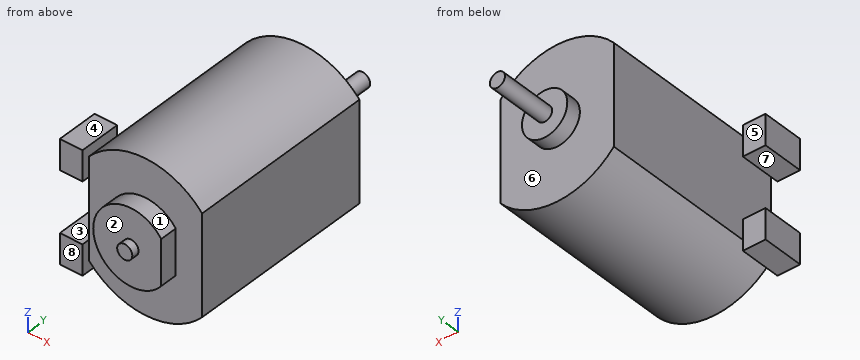
from build123d import *

# Parameters (mm, degrees)
SKETCH_1_R            = 10
EXTRUDE_1_DEPTH       = 25
CUT_EXTRUDE_2_1_REACH = 30.723
SKETCH_2_W            = 2.5
SKETCH_2_H            = 20
SKETCH_3_R            = 3
EXTRUDE_2_DEPTH       = 2
EXTRUDE_START         = -2
SKETCH_4_R            = 1
EXTRUDE_3_DEPTH       = 9.5
EXTRUDE_START_2       = -25
EXTRUDE_4_DEPTH       = 27.3
EXTRUDE_START_3       = 1
SKETCH_6_R            = 1
EXTRUDE_5_DEPTH       = 1
EXTRUDE_6_DEPTH       = 3


with BuildPart() as part:
    # 草图1 → 圆柱凸台-拉伸1 (new body)
    with BuildSketch(Plane(origin=(0, 0, 0), x_dir=(1, 0, 0), z_dir=(0, 1, 0))):
        with Locations(Location((0, 0, 0), (0, 0, 270))):
            Circle(SKETCH_1_R)
    extrude(amount=EXTRUDE_1_DEPTH)

    # 草图2 → 2边切除切除-拉伸1 (cut, up to next)
    with BuildSketch(Plane.XZ, mode=Mode.PRIVATE) as cut_extrude_2_1_sk1:
        with Locations((-8.75, 0)):
            Rectangle(SKETCH_2_W, SKETCH_2_H)
    cut_extrude_2_1_tool1 = extrude(cut_extrude_2_1_sk1.sketch, amount=-CUT_EXTRUDE_2_1_REACH, mode=Mode.PRIVATE) & part.part
    # 草图2 → 2边切除切除-拉伸1 (cut, up to next)
    with BuildSketch(Plane.XZ, mode=Mode.PRIVATE) as cut_extrude_2_1_sk2:
        with Locations((8.75, 0)):
            Rectangle(SKETCH_2_W, SKETCH_2_H)
    cut_extrude_2_1_tool2 = extrude(cut_extrude_2_1_sk2.sketch, amount=-CUT_EXTRUDE_2_1_REACH, mode=Mode.PRIVATE) & part.part
    add(cut_extrude_2_1_tool1.solids().sort_by_distance((-8.75, 0, 0))[0], mode=Mode.SUBTRACT)
    add(cut_extrude_2_1_tool2.solids().sort_by_distance((8.75, 0, 0))[0], mode=Mode.SUBTRACT)

    # 草图3 → 前转凸台-拉伸2 (add)
    with BuildSketch(Plane(origin=(0, 25, 0), x_dir=(1, 0, 0), z_dir=(0, 1, 0))):
        with Locations(Location((0, 0, 0), (0, 0, 270))):
            Circle(SKETCH_3_R)
    extrude(amount=EXTRUDE_2_DEPTH)

    # 草图4 → 前转杆凸台-拉伸3 (add)
    with BuildSketch(Plane(origin=(0, 27, 0), x_dir=(1, 0, 0), z_dir=(0, 1, 0)).offset(EXTRUDE_START)):
        with Locations(Location((0, 0, 0), (0, 0, 270))):
            Circle(SKETCH_4_R)
    extrude(amount=EXTRUDE_3_DEPTH)

    # 草图5 → 后转凸台-拉伸4 (add)
    with BuildSketch(Plane.XZ.offset(EXTRUDE_START_2)):
        with BuildLine():
            Line((4, 3), (4, -3))
            ThreePointArc((4, -3), (-5, 0), (4, 3))
        make_face()
    extrude(amount=EXTRUDE_4_DEPTH)

    # 草图6 → 后转杆凸台-拉伸5 (add)
    with BuildSketch(Plane.XZ.offset(2.3).offset(EXTRUDE_START_3)):
        with Locations(Location((0, 0, 0), (0, 0, 90))):
            Circle(SKETCH_6_R)
    extrude(amount=-EXTRUDE_5_DEPTH)

    # 草图7 → 引线凸台-拉伸6 (add)
    with BuildSketch(Plane.ZY.offset(7.5)):
        Polygon((-8, 3), (-8, 4.5), (-4, 4.5), (-4, 3), (-4, -1), (-8, -1), align=None)
        Polygon((8, 3), (8, -1), (4, -1), (4, 3), (4, 4.5), (8, 4.5), align=None)
    extrude(amount=EXTRUDE_6_DEPTH)


solid = part.part
Input: part model. Units: mm. Frame: model coordinates. Face numbers are marked on the shaded views. A direction names the side the tool comes from. Round coordinates to 2 decimals unless told otherwise and drop trailing zeros. Order: outer loops, then holes, each group sorted by start corner. A loop starts at its lowest first (then second) coordinate and runs counter-clockwise, first axis right, second up. Notation, with made-up numbers: (34.25, 81.5) - (78.25, 81.5) arc R19 ccw to (78.25, 117.5) - close; hole circle Ø8 at (83.25, 50.5). An arc over 180 degrees is marked (long way). Answer as a JSON object with one key per item and string values. Group by question number.
(1) Material intervals for probe 1 along Y at (x, z) = (-4, -1.5); probe 2 along Y at (x, z) = (4.5, 7.75); probe 3 along X at (y, z) = (22.5, 3), sorted ascending. Write a range as from..to.
(2) Cut plane A-A (x = -9). Return loops of the section in (y, z), then the cut area to 3 significant figures.
(3) Pin query (flat end, axial travel): P1, Ø0.9, axis at x = -9, z = 7, coming from the -Y side; P2, Ø8, axis at x = 5.5, y = 28, coming from the -Z side; P3, Ø7, axis at x = 1, z = 1.5, coming from the -Y side; P4, Ø3, axis at x = -5.5, y = 12.5, coming from the -Z side. Return the tip coordinate at first contact, or that it passes through.
(4) Reachability of the marked faces 4, 5, 6, 7 and 8 from +Z, -Z, +X, -X, +Y, -Y: full face, straight path, thin tool, end or side. Return the list, or none.
(5) Draft query along Z for the marked faces 1, 2 and 3. Return one class per face: released by +Z, released by -Z, zero draft, split by the parting line, or undercut.
(6) Cut plane C-C (z = 0). Return loops of the section in (x, y).
(7) Cut plane B-B (y = 2). Return loops of the section in (x, z).
(8) Cut plane D-D (x = 1.75). Return loops of the section in (y, z), then the cut area to 3 significant figures.
Here are the results:
{
 "1": {"probe 1": "y = -2.3..25", "probe 2": "y = 0..25", "probe 3": "x = -7.5..7.5"},
 "2": {"outline": "(-1, -8) - (4.5, -8) - (4.5, -4) - (-1, -4) - close; (-1, 4) - (4.5, 4) - (4.5, 8) - (-1, 8) - close", "area": "44.0 mm^2"},
 "3": {"P1": "stops at y = -1", "P2": "stops at z = -9.58", "P3": "stops at y = -3.3", "P4": "stops at z = -9.17"},
 "4": {"face 4": "+Z, -X, +Y, -Y", "face 5": "+Z, -Z, -X, +Y", "face 6": "+Y", "face 7": "-X, +Y, -Y", "face 8": "+Z, -Z, -X, -Y"},
 "5": {"face 1": "split by the parting line", "face 2": "zero draft", "face 3": "undercut"},
 "6": {"outline": "(-7.5, 0) - (-5, 0) - (-5, -2.3) - (-1, -2.3) - (-1, -3.3) - (1, -3.3) - (1, -2.3) - (4, -2.3) - (4, 0) - (7.5, 0) - (7.5, 25) - (3, 25) - (3, 27) - (1, 27) - (1, 34.5) - (-1, 34.5) - (-1, 27) - (-3, 27) - (-3, 25) - (-7.5, 25) - close"},
 "7": {"outline": "(-10.5, -8) - (-7.5, -8) - (-7.5, -6.61) arc R10 ccw to (7.5, -6.61) - (7.5, 6.61) arc R10 ccw to (-7.5, 6.61) - (-7.5, 8) - (-10.5, 8) - (-10.5, 4) - (-7.5, 4) - (-7.5, -4) - (-10.5, -4) - close"},
 "8": {"outline": "(-2.3, -4.68) - (0, -4.68) - (0, -9.85) - (25, -9.85) - (25, -2.44) - (27, -2.44) - (27, 2.44) - (25, 2.44) - (25, 9.85) - (0, 9.85) - (0, 4.68) - (-2.3, 4.68) - close", "area": "524 mm^2"}
}
